Autodesk Inventor part; units mm, degrees
ref_plane "YZ Plane" through (0, 0, 0) normal (1, 0, 0) x (0, 1, 0)
ref_plane "XZ Plane" through (0, 0, 0) normal (0, 1, 0) x (-1, 0, 0)
ref_plane "XY Plane" through (0, 0, 0) normal (0, 0, 1) x (1, 0, 0)
sketch "BaseProfile" plane through (0, 0, 0) normal (0, 0, 1) x (1, 0, 0)
  circle A0 centre (0, 0) radius 4.925
  circle A1 centre (0, 0) radius 8.925
  line L0 (22.225, -12.8316) -> (0, -25.6632)
  line L1 (0, -25.6632) -> (-22.225, -12.8316)
  line L2 (-22.225, -12.8316) -> (-22.225, 12.8316)
  line L3 (-22.225, 12.8316) -> (0, 25.6632)
  line L4 (0, 25.6632) -> (22.225, 12.8316)
  line L5 (22.225, 12.8316) -> (22.225, -12.8316)
  line L6 (0, -35.9285) -> (0, 35.9285) construction
  line L7 (2.4625, 4.2652) -> (4.925, 0)
  line L8 (4.925, 0) -> (2.4625, -4.2652)
  line L9 (2.4625, -4.2652) -> (-2.4625, -4.2652)
  line L10 (-2.4625, -4.2652) -> (-4.925, 0)
  line L11 (-4.925, 0) -> (-2.4625, 4.2652)
  line L12 (-2.4625, 4.2652) -> (2.4625, 4.2652)
  dimension "d0" = 9.85
  dimension "d1" = 17.85
  dimension "d2" = 44.45
extrude "Extrusion1" add sketch "BaseProfile" against normal blind 7 contours L7 A0 | L8 L9 L10 L11 L12 L7 | A0 L8 | L12 A0 | A0 L9 | L11 A0 | A0 L10 | A1 | L0 L1 L2 L3 L4 L5
extrude "Extrusion2" cut sketch "BaseProfile" against normal blind 1.5 contours L7 A0 | L8 L9 L10 L11 L12 L7 | A0 L8 | L12 A0 | A0 L9 | L11 A0 | A0 L10 | A1
extrude "Extrusion4" cut sketch "BaseProfile" against normal blind 6.35 contours L8 L9 L10 L11 L12 L7
fillet "Fillet1" radius 3.175 6 edges at (-11.1125, -19.2474, -7) (11.1125, -19.2474, -7) (22.225, 0, -7) (-22.225, 0, -7) (-11.1125, 19.2474, -7) (11.1125, 19.2474, -7)
fillet "Fillet2" radius 2 12 edges at (21.2951, -12.2947, -6.0701) (22.225, -12.8316, -1.9125) (21.2951, 12.2947, -6.0701) (22.225, 12.8316, -1.9125) (0, -24.5894, -6.0701) (0, -25.6632, -1.9125) (-21.2951, -12.2947, -6.0701) (-22.225, -12.8316, -1.9125) (-21.2951, 12.2947, -6.0701) (-22.225, 12.8316, -1.9125) (0, 24.5894, -6.0701) (0, 25.6632, -1.9125)
properties part number "pad"
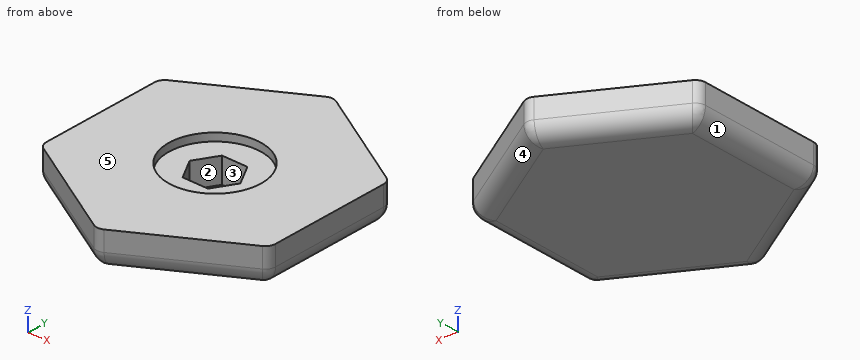
Design review of the part built by this model. Coordinates are the model's own, in mm. Face numbers are marked on the shaded views. A direction names the side the tool comes from. Round coordinates to 2 decimals unless told otherwise and drop trailing zeros. Loops run counter-clockwise (first coordinate to the right, second up) from the corner with the lowest first, then second, coordinate; pieces in that order, holes last. Notation, with made-up numbers: (-32.5, -32) -> (-6.5, -32) arc R25 cw to (-6.5, 1) -> close; hole circle Ø10 at (65, 89.5). An arc over 180 degrees is marked (long way). Use one line per item in the form item = value. Start each with the question number.
Q1. Machinability: for the marked faces 1 and 2, which of the approach directions +Z, -Z, +X, -X, +Y, -Y give a long, thin tool a straight path to every point of the face, cutting with its end or side? Answer none if there is none.
Q2. For pin 1 Ø1 at (y, z) = (20, -2.5) entering from +X (3 decimals); pin 2 Ø14.5 at (x, y) = (0, 0) entering from +Z; pin 3 Ø1.5 at (x, z) = (0.5, -4.5) entering from -Y, all flat-tipped, find the tip position at first contact; note any pin that passes through.
Q3. We need section A-A on z = -0.75. Give the boundary of the cut face in (x, y) (3 decimals), then the cut area to 3 significant figures.
Q4. Draft analysis for pull direction Y (two halves, no side actions). For the marked faces 3, 4 and 5, state which applies: +Y half, -Y half, draft (parallel to the pull), parting line (faces both ways), or undercut.
Q5. Wall thickness on line 1 along Y through (x, z) = (0, -1.1) (3 decimals); line 2 along Y through (x, z) = (5.5, -1); line 3 along Y through (x, z) = (11, -5): over which ranges is each line inside the solid? List them lowest first. Write a range as [from, to].
Q6. We need section B-B on y = -6.5. Give the boundary of the cut face in (x, z) (3 decimals).
Calculated:
q1.face_1 = -Z, -X, +Y, -Y
q1.face_2 = +Z
q2.pin_1 = 10.675
q2.pin_2 = -1.5
q2.pin_3 = -25.35
q3.outline = (-22.225, -11.677) arc R2 ccw to (-21.225, -13.409) -> (-1, -25.086) arc R2 ccw to (1, -25.086) -> (21.225, -13.409) arc R2 ccw to (22.225, -11.677) -> (22.225, 11.677) arc R2 ccw to (21.225, 13.409) -> (1, 25.086) arc R2 ccw to (-1, 25.086) -> (-21.225, 13.409) arc R2 ccw to (-22.225, 11.677) -> close; hole circle Ø17.85 at (0, 0)
q3.area = 1,460 mm²
q4.face_3 = undercut
q4.face_4 = +Y half
q4.face_5 = draft
q5.line_1 = [-25.354, -8.925], [8.925, 25.354]
q5.line_2 = [-22.49, -7.03], [7.03, 22.49]
q5.line_3 = [-19.05, 19.05]
q6.outline = (-22.225, -3.825) arc R3.175 ccw to (-19.05, -7) -> (19.05, -7) arc R3.175 ccw to (22.225, -3.825) -> (22.225, 0) -> (6.116, 0) -> (6.116, -1.5) -> (-6.116, -1.5) -> (-6.116, 0) -> (-22.225, 0) -> close
